Source: CAD feature listing. Evaluate the final solid. Frame: model axes, mm. A direction names the side the tool comes from. Give positions to 0.01 mm unless a question says otherwise; leave off trailing zeros. Order: outer loops, then holes, each group sorted by start corner. A loop starts at its lowest first (then second) coordinate and runs counter-clockwise, first axis right, second up.
```python
from build123d import *

# Parameters (mm, degrees)
F1_DEPTH = 66


# Not quite as in the source:
# - a feature names something its author has since deleted; it is built from what else it names


with BuildPart() as f1:
    # F0 (on Right) → F1 (new body)
    with BuildSketch(Plane.YZ):
        Polygon((-77.412024796, -18.5), (-77.412024796, -24), (87.5, -24), (87.5, -9.63295158), (84.4892114401, -8.5281385109), (84.4892114401, -2.4295686744), (82.965940237, 2.4843649007), (81.7029699683, 3.644410288), (69.5578083396, 6.1807483435), (59.5387034118, 7.6740793884), (49.519598484, 8.5277827457), (49.519598484, 7.9152721193), (49.519598484, 7.5858309865), (48.0495102024, 9.1383457184), (47.6583614945, 7.5858309865), (37.3294272488, 20.848762244), (34.6766483518, 21.9144313596), (32.0238694549, 22.7722087875), (29.0279629678, 23.3218624368), (26.0279629678, 23.7739541456), (23.0279629678, 24), (-13.387337327, 24), (-14.9341821671, 23.5386695713), (-15.2199724689, 23.2877042145), (-16.9720370322, 7.4994475581), (-83.4866687655, 7.4994475581), (-83.4866687655, -10.5200763792), (-87.5, -10.5200763792), (-87.5, -16.75), (-84.6275396049, -17.125), (-84.412024796, -17.5), (-81.795014441, -17.5), (-81.412024796, -18), align=None)
    extrude(amount=-F1_DEPTH)


solid = f1.part
```
1) Pin query (flat end, axial travel): pin 1 (8 mm diameter, centred on x = -44, z = 14.5, fed in from +Y); pin 2 (3 mm diameter, centred on x = -27, y = -60, fed in from +Z); pin 3 (6 mm diameter, centred on x = -32.5, z = -22, fed in from -Y). Return the tip coordinate at first contact, or that it passes through.
Report:
pin 1: stops at y = 45.39
pin 2: stops at z = 7.5
pin 3: stops at y = -77.41
2) Reachability of faces 1 (the flat face through (-33, -85, -10.52)), 2 (the flat face through (-33, -77.412, -21)), 3 (the flat face through (-66, -1, -5)), 4 (the flat face through (-33, 84.489, -6)) from +Z, -Z, +X, -X, +Y, -Y: full face, straight path, thin tool, end or side. Return the list, or none.
Report:
face 1: +Z, +X, -X, -Y
face 2: -Z, +X, -X, -Y
face 3: +Z, -Z, -X, +Y, -Y
face 4: +Z, +X, -X, +Y
3) Section query C-C, the plane z = 17.5. Return the cut outline in (x, y), and give its area (3 significant figures).
Report:
outline: (-66, -15.86) - (0, -15.86) - (0, 39.94) - (-66, 39.94) - close
area: 3,680 mm2
4) Section query B-B, the plane y = -43.5. Return the cut outline in (x, z), and give its area (3 significant figures).
Report:
outline: (-66, -24) - (0, -24) - (0, 7.5) - (-66, 7.5) - close
area: 2,080 mm2
5) Material intervals for L1, parallel to Z at x = -33, y = 59.5; L2, parallel to Y at x = -33, z = -4.5; L3, parallel to Z at x = -25, y = -59.5, sorted ascending.
Report:
L1: z = -24 to 7.68
L2: y = -83.49 to 84.49
L3: z = -24 to 7.5
